```python
from build123d import *

# Parameters (mm, degrees)
BOSS_EXTRUDE1_DEPTH   = 10
CUT_EXTRUDE6_DEPTH    = 29.232073959
BOSS_EXTRUDE4_DEPTH   = 1.9
CUT_EXTRUDE7_DEPTH    = 1.1
BOSS_EXTRUDE5_START   = -10
SKETCH31_W            = 6.6
SKETCH31_H            = 20.8
BOSS_EXTRUDE5_DEPTH   = 10
SKETCH32_W            = 1.175
SKETCH32_H            = 20.8
SKETCH32_W_2          = 1.425
BOSS_EXTRUDE6_DEPTH   = 1.2
SKETCH33_W            = 3
SKETCH33_H            = 10
BOSS_EXTRUDE7_DEPTH   = 1.65
SKETCH34_W            = 3
SKETCH34_H            = 10
BOSS_EXTRUDE8_DEPTH   = 1.65
BODY_MOVE_COPY1_ANGLE = 180


with BuildPart() as part:
    # Sketch1 → Boss-Extrude1 (new body)
    with BuildSketch(Plane.XY):
        with BuildLine():
            Line((7.490021902, 0), (21.300000001, 0))
            Line((21.300000001, 0), (21.300000001, 4.05))
            Line((21.300000001, 4.05), (9.555596341, 4.05))
            ThreePointArc((9.555596341, 4.05), (3.627957458, 7.8), (9.555596341, 11.55))
            Line((9.555596341, 11.55), (21.300000001, 11.55))
            Line((21.300000001, 11.55), (21.300000001, 15.6))
            Line((21.300000001, 15.6), (7.911262801, 15.6))
            ThreePointArc((7.911262801, 15.6), (0.108419667, 8.005009917), (7.490021902, 0))
        make_face()
    extrude(amount=-BOSS_EXTRUDE1_DEPTH)

    # Sketch19 → Cut-Extrude6 (cut, through all)
    with BuildSketch(Plane.XZ):
        with BuildLine():
            Line((15.975079943, -6.392558475), (15.000000001, -7.075316801))
            Line((15.000000001, -7.075316801), (14.024920059, -6.392558475))
            ThreePointArc((14.024920059, -6.392558475), (15.000000001, -3.3), (15.975079943, -6.392558475))
        make_face()
    extrude(amount=-CUT_EXTRUDE6_DEPTH, mode=Mode.SUBTRACT)

    # Sketch21 → Boss-Extrude4 (add)
    with BuildSketch(Plane(origin=(0, 15.6, 0), x_dir=(1, 0, 0), z_dir=(0, 1, 0))):
        Polygon((20.773502693, 5), (17.886751347, 10), (12.113248655, 10), (9.226497309, 5), (12.113248655, 0), (17.886751347, 0), align=None)
        Polygon((13.267949194, 8), (11.535898386, 5), (13.267949194, 2), (16.732050809, 2), (18.464101616, 5), (16.732050809, 8), align=None, mode=Mode.SUBTRACT)
    extrude(amount=BOSS_EXTRUDE4_DEPTH)

    # Sketch22 → Cut-Extrude7 (cut)
    with BuildSketch(Plane(origin=(0, 15.6, 0), x_dir=(1, 0, 0), z_dir=(0, 1, 0))):
        Polygon((16.732050809, 8), (13.267949194, 8), (11.535898386, 5), (13.267949194, 2), (16.732050809, 2), (18.464101616, 5), align=None)
    extrude(amount=-CUT_EXTRUDE7_DEPTH, mode=Mode.SUBTRACT)

    # Sketch31 → Boss-Extrude5 (add)
    with BuildSketch(Plane(origin=(0, 0, -10), x_dir=(-1, 0, 0), z_dir=(0, 0, -1)).offset(BOSS_EXTRUDE5_START)):
        with BuildLine():
            Line((1.642634889, 18.194312696), (1.642634889, 16.194312696))
            ThreePointArc((1.642634889, 16.194312696), (0.002167009, 13.578091054), (-3.067375979, 13.915220696))
            ThreePointArc((-3.067375979, 13.915220696), (-0.105575497, 7.794312696), (-3.067375979, 1.673404696))
            ThreePointArc((-3.067375979, 1.673404696), (0.002167009, 2.010534337), (1.642634889, -0.605687304))
            Line((1.642634889, -0.605687304), (1.642634889, -2.608681933))
            ThreePointArc((1.642634889, -2.608681933), (2.210176801, -3.836976077), (3.512045594, -4.205687304))
            Line((3.512045594, -4.205687304), (9.862045594, -4.205687304))
            ThreePointArc((9.862045594, -4.205687304), (10.993416444, -3.737058154), (11.462045594, -2.605687304))
            Line((11.462045594, -2.605687304), (11.462045594, 18.194312696))
            ThreePointArc((11.462045594, 18.194312696), (10.993416444, 19.325683546), (9.862045594, 19.794312696))
            Line((9.862045594, 19.794312696), (3.512027658, 19.794312696))
            ThreePointArc((3.512027658, 19.794312696), (2.209033865, 19.424620515), (1.642634889, 18.194312696))
        make_face()
        with Locations((6.562045594, 7.794312696)):
            Rectangle(SKETCH31_W, SKETCH31_H, mode=Mode.SUBTRACT)
    extrude(amount=BOSS_EXTRUDE5_DEPTH)

    # Sketch32 → Boss-Extrude6 (add)
    with BuildSketch(Plane.XY):
        with Locations((-3.849545594, 7.794312696)):
            Rectangle(SKETCH32_W, SKETCH32_H)
        with Locations((-9.149545594, 7.794312696)):
            Rectangle(SKETCH32_W_2, SKETCH32_H)
    extrude(amount=-BOSS_EXTRUDE6_DEPTH)

    # Sketch33 → Boss-Extrude7 (add)
    with BuildSketch(Plane.XZ.offset(-11.55)):
        with Locations((19.800000001, -5)):
            Rectangle(SKETCH33_W, SKETCH33_H)
    extrude(amount=BOSS_EXTRUDE7_DEPTH)

    # Sketch34 → Boss-Extrude8 (add)
    with BuildSketch(Plane(origin=(0, 4.05, 0), x_dir=(1, 0, 0), z_dir=(0, 1, 0))):
        with Locations((19.800000001, 5)):
            Rectangle(SKETCH34_W, SKETCH34_H)
    extrude(amount=BOSS_EXTRUDE8_DEPTH)


with BuildPart() as part_1:
    # Body-Move/Copy1: read off the stored shape, not the designer's step
    # Body-Move/Copy1: moved
    add(part.part.moved(Location((-21.9272776, -16.282285, 0))).rotate(Axis((0, 0, 0), (0.7071067812, -0.7071067812, 0)), BODY_MOVE_COPY1_ANGLE))


solid = part_1.part
```
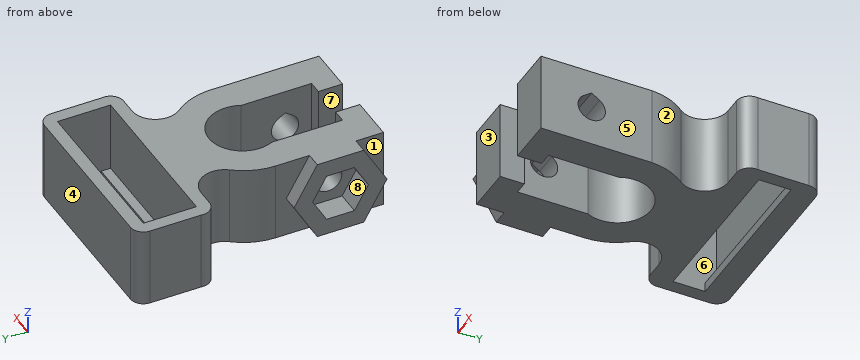
Check sheet for the modelled part. Datum: model origin and axes. Units: mm. Face numbers are marked on the shaded views. A direction names the side the tool comes from. Give positions to 0.01 mm unless a question says otherwise; leave off trailing zeros. Loops run counter-clockwise (first coordinate to the right, second up) from the corner with the lowest first, then second, coordinate; pieces in that order, holes last. Notation, with made-up numbers: M 43.25,-9.5 L 85.25,-9.5 A13 cw 85.25,9.5 Z; hole C 53.25,60.25 d10. An arc over 180 degrees is marked long. Answer in a Markdown table with one row per item.
1) Cross-section at A-A (x = -0.25). Enter the section's corners in (y, z).
Solutions:
| item | result |
|---|---|
| outline | M 1.15,5 L 4.04,0 L 9.81,0 L 12.7,5 L 9.81,10 L 4.04,10 Z; M 23.57,0 L 26.36,0 L 26.36,1.2 L 25.19,1.2 L 25.19,10 L 23.57,10 Z; M 30.36,0 L 33.39,0 L 33.39,10 L 31.79,10 L 31.79,1.2 L 30.36,1.2 Z; hole M 3.46,5 L 5.2,2 L 8.66,2 L 10.39,5 L 8.66,8 L 5.2,8 Z |
2) Thickness scan on line 1 (Y direction, x = 13.7, z = 5); line 2 (Y direction, x = -0.75, z = 6.5); line 3 (Y direction, x = 17, z = 5.5). Record the ranges inside material, lowest first.
Solutions:
| item | result |
|---|---|
| line 1 | y = 0.63 to 5.23, 8.63 to 25.19, 31.79 to 33.39 |
| line 2 | y = 2.02 to 4.33, 9.53 to 11.83, 23.57 to 25.19, 31.79 to 33.39 |
| line 3 | y = 23.57 to 25.19, 31.79 to 33.39 |
3) Cross-section at D-D (x = 7). Enter the section's corners in (y, z).
Solutions:
| item | result |
|---|---|
| outline | M 18.03,0 L 26.36,0 L 26.36,1.2 L 25.19,1.2 L 25.19,10 L 18.03,10 Z; M 30.36,0 L 33.39,0 L 33.39,10 L 31.79,10 L 31.79,1.2 L 30.36,1.2 Z |
4) Mould release check, pull along Y, two halves, no side actions. Record for the marked faces 1, 2, 3 and 4: released by +Y, released by -Y, zero draft, split by the parting line, or undercut.
Solutions:
| item | result |
|---|---|
| face 1 | zero draft |
| face 2 | undercut |
| face 3 | released by -Y |
| face 4 | released by +Y |
5) Depth check by flat-ended pin: pin 1 (2 mm diameter, centred on y = 12, z = 7, fed in from -X); pin 2 (2 mm diameter, centred on y = 6.93, z = 5, fed in from -X); pin 3 (0.6 mm diameter, centred on x = 8.5, y = 26, fed in from +Z); pin 4 (3 mm diameter, centred on y = 30, z = 6.5, fed in from -X). Enter the tip coordinate at first touch or a pass-through.
Solutions:
| item | result |
|---|---|
| pin 1 | stops at x = -1.22 |
| pin 2 | passes through |
| pin 3 | stops at z = 1.2 |
| pin 4 | stops at x = -3.51 |
6) Tool access check on the marked faces 5, 6, 7 and 8. Record the directions out of +Z, -Z, +X, -X, +Y, -Y that give a thin tool (end or side, any length) a straight path to the whole face; none if there is none.
Solutions:
| item | result |
|---|---|
| face 5 | +Z, -Z, +X, -Y |
| face 6 | +Z |
| face 7 | +Z, -Z, -Y |
| face 8 | -X |
7) Cross-section at C-C (x = 3.75). Enter the section's corners in (y, z).
Solutions:
| item | result |
|---|---|
| outline | M 0.63,0 L 26.36,0 L 26.36,1.2 L 25.19,1.2 L 25.19,10 L 0.63,10 Z; M 30.36,0 L 33.39,0 L 33.39,10 L 31.79,10 L 31.79,1.2 L 30.36,1.2 Z; hole M 5.95,6.39 A1.7 ccw long 7.9,6.39 L 6.93,7.08 Z |
8) Cross-section at B-B (y = 29.5). Enter the section's corners in (x, z).
Solutions:
| item | result |
|---|---|
| outline | M -3.51,0 L -1.91,0 L -1.91,10 L -3.51,10 Z; M 18.89,0 L 20.49,0 L 20.49,10 L 18.89,10 Z |
